Solid Edge part; units mm, degrees
sketch "Sketch1" plane through (0, 0, 0) normal (0, 0, 1) x (1, 0, 0)
  line L0 (7.9, 4) -> (-7.9, 4)
  line L1 (-7.9, 4) -> (-7.9, -4)
  line L2 (-7.9, -4) -> (7.9, -4)
  line L3 (7.9, -4) -> (7.9, 4)
extrude "Protrusion1" add sketch "Sketch1" against normal blind 3.2
sketch "Sketch2" plane through (0, 0, -3.2) normal (0, 0, -1) x (0, 1, 0)
  line L0 (2.5, -6.5) -> (2.5, 6.5)
  line L1 (2.5, 6.5) -> (-2.5, 6.5)
  line L2 (-2.5, 6.5) -> (-2.5, -6.5)
  line L3 (-2.5, -6.5) -> (2.5, -6.5)
  circle A0 centre (0, 0) radius 1.4
  circle A1 centre (0, 0) radius 0.8
extrude "ExtrudedCutout_1" cut sketch "Sketch2" against normal blind 2
sketch "Sketch3" plane through (0, 0, 0) normal (0, 0, 1) x (0, -1, 0)
  circle A0 centre (0, 4) radius 2.4
  circle A1 centre (0, -4) radius 2.4
extrude "ExtrudedProtrusion_2" add sketch "Sketch3" along normal blind 1.8
The listing builds one solid part. Answer for the finished solid, in the listing's coordinates (mm). A direction names the side the tool comes from. Coordinates: 2 decimals unless noted, no trailing zeros. Write each loop counter-clockwise with the first axis right and the second up, starting at its lowest first coordinate (ties: lowest second). Pieces come first, ordered by that corner, then holes. Notation, with made-up numbers: (-5.5, 6.5) - (-0.5, 6.5) arc R25 cw to (-0.5, 45.5) - close; hole circle Ø5 at (20, 65.25). An arc over 180 degrees is marked (long way). One line per item, written item: value.
1) Consider line 1 along X through (y, z) = (0, -1.6); line 2 along X through (y, z) = (1.75, -2.55); line 3 along Y through (x, z) = (-1, -1.35). Determine where each line is inside the solid, lowest interval first. Write a range as from..to.
Geometry check:
line 1: x = -7.9..-6.5, -1.4..-0.8, 0.8..1.4, 6.5..7.9
line 2: x = -7.9..-6.5, 6.5..7.9
line 3: y = -4..-2.5, -0.98..0.98, 2.5..4
2) Find section D-D (z = 1.55). Give the vertices of the cut face in (x, y).
Geometry check:
outline: circle Ø4.8 at (-4, 0); circle Ø4.8 at (4, 0)
3) For a pull along X with two mould halves and no side action, classify faces 4 (the flat face through (4, 0, 1.8)), 5 (the flat face through (0, 0, 0)), 6 (the flat face through (-7.9, 0, -2)) as pulls with the +X half, pulls with the -X half, needs draft (parallel to the pull), parting line crosses it, or undercut.
Geometry check:
face 4: needs draft
face 5: undercut
face 6: pulls with the -X half
4) Find section C-C (x = -4). Give the vertices of the cut face in (y, z), and give its area (3 significant figures).
Geometry check:
outline: (-4, -3.2) - (-2.5, -3.2) - (-2.5, -1.2) - (2.5, -1.2) - (2.5, -3.2) - (4, -3.2) - (4, 0) - (2.4, 0) - (2.4, 1.8) - (-2.4, 1.8) - (-2.4, 0) - (-4, 0) - close
area: 24.2 mm2
5) Find section B-B (y = 0). Give the vertices of the cut face in (x, z), and give its area (3 significant figures).
Geometry check:
outline: (-7.9, -3.2) - (-6.5, -3.2) - (-6.5, -1.2) - (-1.4, -1.2) - (-1.4, -3.2) - (-0.8, -3.2) - (-0.8, -1.2) - (0.8, -1.2) - (0.8, -3.2) - (1.4, -3.2) - (1.4, -1.2) - (6.5, -1.2) - (6.5, -3.2) - (7.9, -3.2) - (7.9, 0) - (6.4, 0) - (6.4, 1.8) - (1.6, 1.8) - (1.6, 0) - (-1.6, 0) - (-1.6, 1.8) - (-6.4, 1.8) - (-6.4, 0) - (-7.9, 0) - close
area: 44.2 mm2
6) Each of these flat-tipped pins is pushed along its axis until it touches: pin 1 Ø0.5 at (x, y) = (-0.5, 0) entering from -Z; pin 2 Ø1.5 at (x, z) = (-4.5, 1) entering from -Y. Where does it stop, or does it pass through?
Geometry check:
pin 1: stops at z = -1.2
pin 2: stops at y = -2.4
7) Find section A-A (z = -2.85). Give the vertices of the cut face in (x, y).
Geometry check:
outline: (-7.9, -4) - (7.9, -4) - (7.9, 4) - (-7.9, 4) - close; circle Ø2.8 at (0, 0); hole (-6.5, -2.5) - (6.5, -2.5) - (6.5, 2.5) - (-6.5, 2.5) - close; hole circle Ø1.6 at (0, 0)
8) A tool of negligible diameter and unlimited length cuts with its end or side. For faces 1 (the cylindrical face through (-6.024, -1.29, 0.887)), 2 (the flat face through (0, -2.5, -2)), 3 (the flat face through (0, -4, -2)), from which of +Z, -Z, +X, -X, +Y, -Y can it reach the whole face along a straight path? Write none if from no direction.
Geometry check:
face 1: +Z
face 2: -Z
face 3: +Z, -Z, +X, -X, -Y
